Autodesk Inventor part; units mm, degrees
ref_plane "YZ Plane" through (0, 0, 0) normal (1, 0, 0) x (0, 1, 0)
ref_plane "XZ Plane" through (0, 0, 0) normal (0, 1, 0) x (-1, 0, 0)
ref_plane "XY Plane" through (0, 0, 0) normal (0, 0, 1) x (1, 0, 0)
sketch "Sketch1" plane through (0, 0, 0) normal (0, 1, 0) x (-1, 0, 0)
  line L0 (-36.7054, 45.2992) -> (63.2946, 45.2992)
  line L1 (63.2946, 45.2992) -> (63.2946, -54.7008)
  line L2 (63.2946, -54.7008) -> (-36.7054, -54.7008)
  line L3 (-36.7054, -54.7008) -> (-36.7054, 45.2992)
  line L4 (73.2946, -74.7008) -> (-46.7054, -74.7008)
  line L5 (-46.7054, -74.7008) -> (-46.7054, 65.2992)
  line L6 (-46.7054, 65.2992) -> (73.2946, 65.2992)
  line L7 (73.2946, 65.2992) -> (73.2946, -74.7008)
  point P0 (0, 0)
  dimension "d0" = 100
  dimension "d1" = 100
  dimension "d2" = 120
  dimension "d3" = 140
  dimension "d4" = 20
  dimension "d5" = 10
extrude "Plate1" add sketch "Sketch1" along normal blind 1.5875
sketch "Sketch2" plane through (45.1179, 0, -74.7008) normal (1, 0, 0) x (0, 1, 0)
  line L0 (0, 140) -> (0, 0)
  line L1 (0, 0) -> (40, 0)
  line L2 (40, 0) -> (40, 140)
  line L3 (40, 140) -> (0, 140)
edge flange "Flange1" height 40 angle 90 thickness 1.5875 bend radius 1.5875 thickness toward (1, 0, 0) relief tear relief width 1.5875 relief depth 0.7937 edges at (46.7054, 1.5875, -4.7008) wall of the first edge with corners at (45.1179, 0, 65.2992) (45.1179, 0, -74.7008) (45.1179, 40, -74.7008) (45.1179, 40, 65.2992)
bend "Bend1"
corner "Corner1"
sketch "Sketch3" plane through (-71.7071, 0, 65.2992) normal (-1, 0, 0) x (0, -1, 0)
  line L0 (0, -140) -> (0, 0)
  line L1 (0, 0) -> (-40, 0)
  line L2 (-40, 0) -> (-40, -140)
  line L3 (-40, -140) -> (0, -140)
edge flange "Flange2" height 40 angle 90 thickness 1.5875 bend radius 1.5875 thickness toward (-1, 0, 0) relief tear relief width 1.5875 relief depth 0.7937 edges at (-73.2946, 1.5875, -4.7008) wall of the first edge with corners at (-71.7071, 0, -74.7008) (-71.7071, 0, 65.2992) (-71.7071, 40, 65.2992) (-71.7071, 40, -74.7008)
bend "Bend2"
corner "Corner2"
sketch "Sketch4" plane through (-73.2946, 38.4125, 65.2992) normal (0, 1, 0) x (-1, 0, 0)
  line L0 (0, -140) -> (0, 0)
  line L1 (0, 0) -> (-10, 0)
  line L2 (-10, 0) -> (-10, -140)
  line L3 (-10, -140) -> (0, -140)
edge flange "Flange3" height 10 angle 90 thickness 1.5875 bend radius 1.5875 thickness toward (0, 1, 0) relief tear relief width 1.5875 relief depth 0.7937 edges at (-71.7071, 40, -4.7008) wall of the first edge with corners at (-73.2946, 38.4125, -74.7008) (-73.2946, 38.4125, 65.2992) (-63.2946, 38.4125, 65.2992) (-63.2946, 38.4125, -74.7008)
bend "Bend3"
corner "Corner3"
sketch "Sketch5" plane through (46.7054, 38.4125, -74.7008) normal (0, 1, 0) x (-1, 0, 0)
  line L0 (0, 140) -> (0, 0)
  line L1 (0, 0) -> (10, 0)
  line L2 (10, 0) -> (10, 140)
  line L3 (10, 140) -> (0, 140)
edge flange "Flange4" height 10 angle 90 thickness 1.5875 bend radius 1.5875 thickness toward (0, 1, 0) relief tear relief width 1.5875 relief depth 0.7937 edges at (45.1179, 40, -4.7008) wall of the first edge with corners at (46.7054, 38.4125, 65.2992) (46.7054, 38.4125, -74.7008) (36.7054, 38.4125, -74.7008) (36.7054, 38.4125, 65.2992)
bend "Bend4"
corner "Corner4"
equation "\"d7\" = BendReliefWidth"
equation "\"d8\" = BendReliefDepth"
equation "\"d9\" = MinimumRemnant"
equation "\"d10\" = BendRadius"
equation "\"d13\" = BendRadius"
equation "\"d14\" = CornerReliefSize"
equation "\"d15\" = GapSize"
equation "\"d16\" = JacobiRadiusSize"
equation "\"d17\" = BendReliefWidth"
equation "\"d18\" = BendReliefDepth"
equation "\"d19\" = MinimumRemnant"
equation "\"d20\" = BendRadius"
equation "\"d23\" = BendRadius"
equation "\"d24\" = CornerReliefSize"
equation "\"d25\" = GapSize"
equation "\"d26\" = JacobiRadiusSize"
equation "\"d27\" = BendReliefWidth"
equation "\"d28\" = BendReliefDepth"
equation "\"d29\" = MinimumRemnant"
equation "\"d30\" = BendRadius"
equation "\"d33\" = BendRadius"
equation "\"d34\" = CornerReliefSize"
equation "\"d35\" = GapSize"
equation "\"d36\" = JacobiRadiusSize"
equation "\"d37\" = BendReliefWidth"
equation "\"d38\" = BendReliefDepth"
equation "\"d39\" = MinimumRemnant"
equation "\"d40\" = BendRadius"
equation "\"d43\" = BendRadius"
equation "\"d44\" = CornerReliefSize"
equation "\"d45\" = GapSize"
equation "\"d46\" = JacobiRadiusSize"
equation "\"BendRadius\" = Thickness"
equation "\"BendReliefWidth\" = Thickness"
equation "\"BendReliefDepth\" = 0.5 * Thickness"
equation "\"CornerReliefSize\" = 4 * Thickness"
equation "\"MinimumRemnant\" = 2 * Thickness"
equation "\"TransitionRadius\" = BendRadius"
equation "\"JacobiRadiusSize\" = BendRadius"
equation "\"GapSize\" = Thickness"
equation "\"d6\" = BendRadius"
properties part number "DishFanMetal"
Geometry check sheet. Reference: the model listing, model coordinates, mm. A direction names the side the tool comes from. Round coordinates to 2 decimals unless told otherwise and drop trailing zeros. Order: outer loops, then holes, each group sorted by start corner. A loop starts at its lowest first (then second) coordinate and runs counter-clockwise, first axis right, second up. Notation, with made-up numbers: M 60,-4 L 87,-4 A20 cw 87,32 Z; hole C 27.25,-12 d4. An arc over 180 degrees is marked long. Write item = value, one per line.
Q1. Section check C-C (x = -53). Enter the section's corners in (y, z).
Answer block:
outline = M 0,-74.7 L 1.59,-74.7 L 1.59,-54.7 L 0,-54.7 Z; M 0,45.3 L 1.59,45.3 L 1.59,65.3 L 0,65.3 Z
Q2. Scan lines: line 1 (X direction, y = 25, z = -17); line 2 (Y direction, x = -53, z = 59). Record each from-to range of solid material in increasing order.
Answer block:
line_1 = -73.29 to -71.71, 45.12 to 46.71
line_2 = 0 to 1.59
Q3. Depth check by flat-ended pin: pin 1 Ø0.5 at (y, z) = (39, -30.5) entering from -X; pin 2 Ø1.7 at (y, z) = (1, -24) entering from -X; pin 3 Ø3 at (x, z) = (-14, -60.5) entering from +Y. Enter the tip coordinate at first touch or a pass-through.
Answer block:
pin_1 = -72.64
pin_2 = -73
pin_3 = 1.59
Q4. Release check for a two-part mould opening along X. For faces 1 (the flat face through (40, 40, -6)), 2 (the flat face through (46.705, 20, -6)), 3 (the flat face through (45.118, 20, -6)) record: released by +X, released by -X, zero draft, split by the parting line, or undercut.
Answer block:
face_1 = zero draft
face_2 = released by +X
face_3 = undercut
Q5. Set-up check for faces 4 (the flat face through (37, 1.588, -10)), 5 (the flat face through (-73.295, 20, -4)): record each of +Z, -Z, +X, -X, +Y, -Y from which the full face is reachable in a straight line by a thin tool's end or side.
Answer block:
face_4 = +Z, -Z
face_5 = +Z, -Z, -X, +Y, -Y
Q6. Section check A-A (y = 33). Enter the section's corners in (x, z), plus the area to 4 significant figures.
Answer block:
outline = M -73.29,-74.7 L -71.71,-74.7 L -71.71,65.3 L -73.29,65.3 Z; M 45.12,-74.7 L 46.71,-74.7 L 46.71,65.3 L 45.12,65.3 Z
area = 444.5 mm^2
